Source: three-view drawing plus pictorial views. Frame: mm from the lowest corner of the part. A direction names the side the tool comes from. Round coordinates to 2 decimals unless told otherwise and drop trailing zeros. Write each loop counter-clockwise with the first axis right and the second up, starting at its lowest first coordinate (ties: lowest second). Pieces come first, ordered by that corner, then holes.
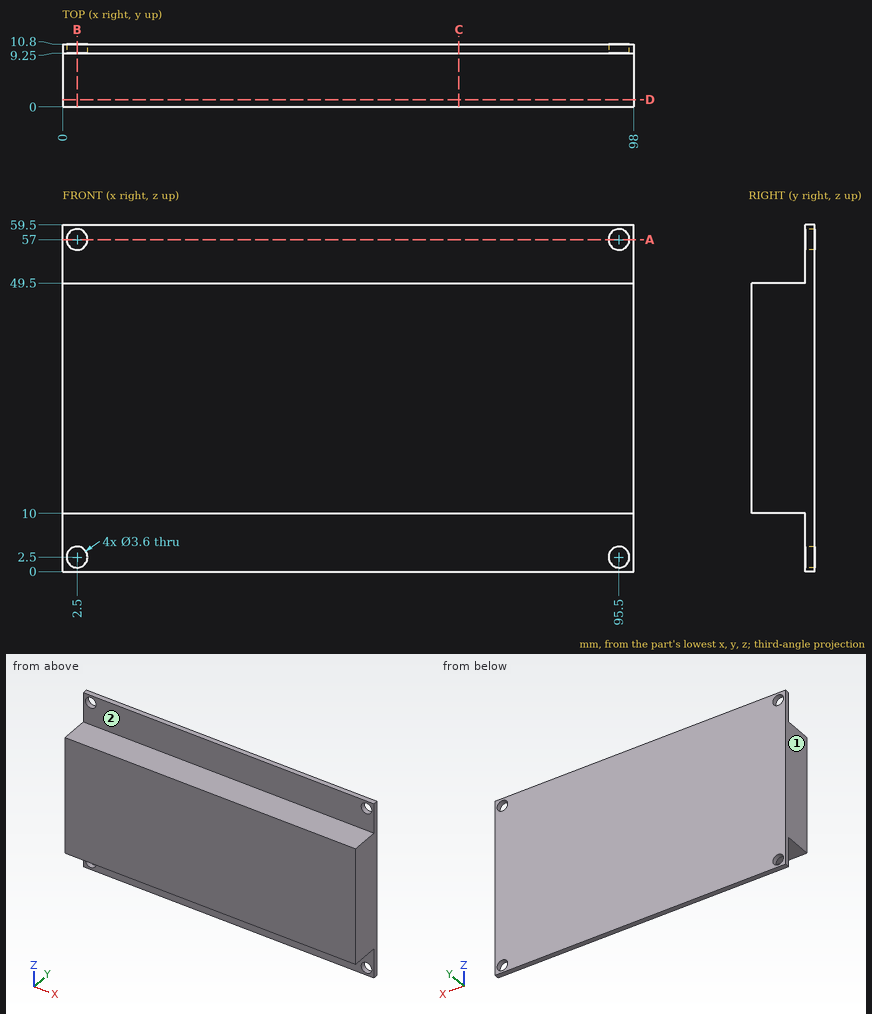
1) Section D-D on y = 1.25. Output: boundary loops of the cut face in (x, z), plus the area to 3 significant figures.
2) Section B-B on x = 2.5. Output: boundary loops of the cut face in (y, z).
3) Section C-C on x = 68. Output: boundary loops of the cut face in (y, z).
4) Reachability of the marked faces 1 and 2 from +Z, -Z, +X, -X, +Y, -Y: full face, straight path, thin tool, end or side. Return the list, or none.
5) Line query: probe 1 along Z at (x, y) = (2.5, 10.25); probe 2 along Z at (x, y) = (74, 1.5); probe 3 along Y at (x, z) = (19, 7.5). Output: solid intervals per line, ascending.
6) Section A-A on z = 57. Output: boundary loops of the cut face in (x, y), plus the area to 3 significant figures.
7) First-contact query: P1, Ø4, axis at x = 2.5, z = 57, coming from the -Y side; P2, Ø1, axis at x = 62.5, y = 8.5, coming from the +Z side; P3, Ø3, axis at x = 2.5, z = 2.5, coming from the +Y side. Flat tips, straight axial feed; report the tip coordinate or a pass-through.
Filled in:
1. outline: (0, 10) - (98, 10) - (98, 49.5) - (0, 49.5) - close
1. area: 3,870 mm2
2. outline: (0, 10) - (9.25, 10) - (9.25, 4.3) - (10.8, 4.3) - (10.8, 55.2) - (9.25, 55.2) - (9.25, 49.5) - (0, 49.5) - close; (9.25, 0) - (10.8, 0) - (10.8, 0.7) - (9.25, 0.7) - close; (9.25, 58.8) - (10.8, 58.8) - (10.8, 59.5) - (9.25, 59.5) - close
3. outline: (0, 10) - (9.25, 10) - (9.25, 0) - (10.8, 0) - (10.8, 59.5) - (9.25, 59.5) - (9.25, 49.5) - (0, 49.5) - close
4. face 1: +Z, -Z, -X, +Y, -Y
4. face 2: +Z, +X, -X, -Y
5. probe 1: z = 0 to 0.7, 4.3 to 55.2, 58.8 to 59.5
5. probe 2: z = 10 to 49.5
5. probe 3: y = 9.25 to 10.8
6. outline: (0, 9.25) - (0.7, 9.25) - (0.7, 10.8) - (0, 10.8) - close; (4.3, 9.25) - (93.7, 9.25) - (93.7, 10.8) - (4.3, 10.8) - close; (97.3, 9.25) - (98, 9.25) - (98, 10.8) - (97.3, 10.8) - close
6. area: 141 mm2
7. P1: stops at y = 9.25
7. P2: stops at z = 49.5
7. P3: passes through
